Part print with two shaded views. Sizes in mm from the minimum x, y, z corner. Round coordinates to 2 decimals unless told otherwise and drop trailing zeros. Order: outer loops, then holes, each group sorted by start corner. A loop starts at its lowest first (then second) coordinate and runs counter-clockwise, first axis right, second up. Notation, with made-up numbers: (-38.75, 53) - (-2.75, 53) arc R11 ccw to (-2.75, 69) - close; hole circle Ø5 at (-7, -4). An arc over 180 degrees is marked (long way). Use one line per item in the form item = value.
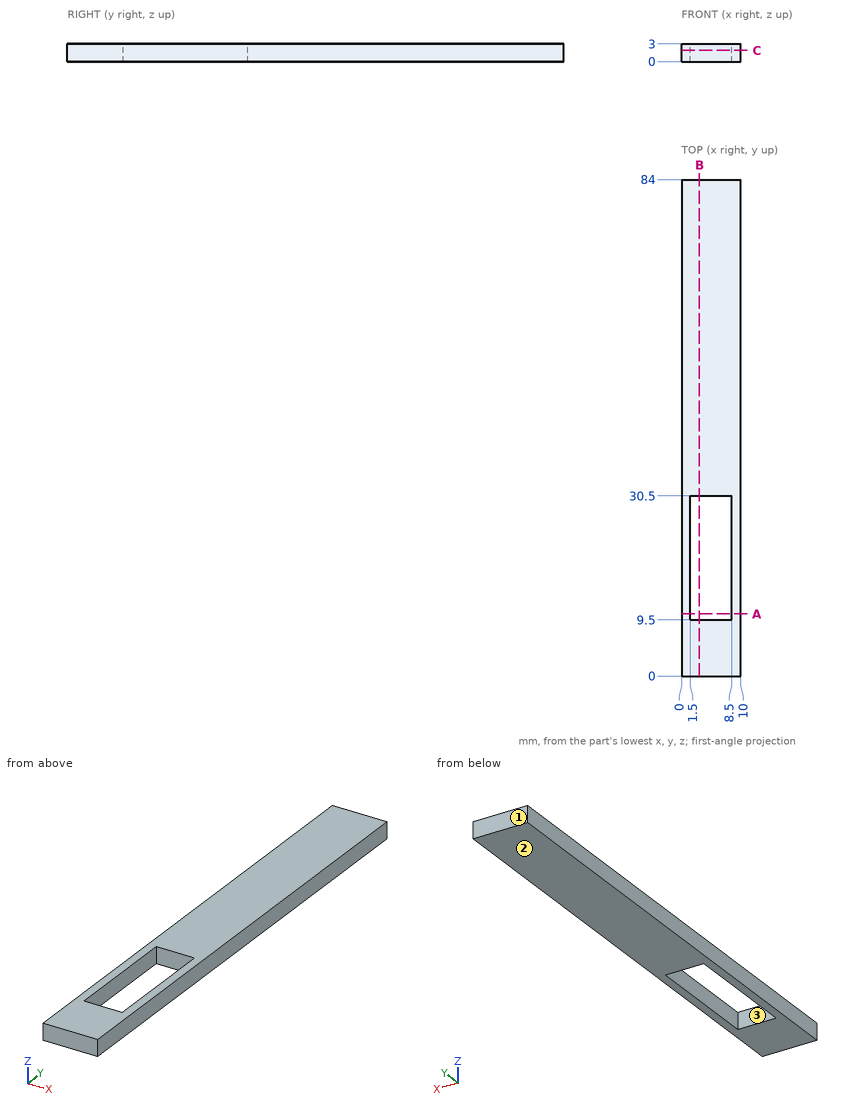
(1) Pin check, flat tip, straight feed: pin 1 (1.5 mm diameter, centred on y = 22, z = 0.5, fed in from -X). Stop position of the tip, or through.
Report:
pin_1 = 0
(2) Slice it at A-A on y = 10.5. Give the cut face in (x, z).
Report:
outline = (0, 0) - (1.5, 0) - (1.5, 3) - (0, 3) - close; (8.5, 0) - (10, 0) - (10, 3) - (8.5, 3) - close
(3) Pull direction Y, two halves, no side cores. Call the marked faces 1, 2 and 3: released by +Y, released by -Y, zero draft, split by the parting line, or undercut.
Report:
face_1 = released by +Y
face_2 = zero draft
face_3 = undercut
(4) Slice it at B-B on x = 3. Give the cut face in (y, z).
Report:
outline = (0, 0) - (9.5, 0) - (9.5, 3) - (0, 3) - close; (30.5, 0) - (84, 0) - (84, 3) - (30.5, 3) - close
(5) Probe probe 1 along Y at (x, z) = (6.5, 1.85); probe 2 along X at (y, z) = (16, 0.6). List the from-to ranges inside material, lowest first. Write a range as [from, to].
Report:
probe_1 = [0, 9.5], [30.5, 84]
probe_2 = [0, 1.5], [8.5, 10]
(6) Slice it at C-C on z = 1.9. Give the cut face in (x, y), then the cut area to 3 significant figures.
Report:
outline = (0, 0) - (10, 0) - (10, 84) - (0, 84) - close; hole (1.5, 9.5) - (8.5, 9.5) - (8.5, 30.5) - (1.5, 30.5) - close
area = 693 mm2
